The model under review builds one solid part; all positions refer to its coordinate system, in mm. A direction names the side the tool comes from. Coordinates: 2 decimals unless noted, no trailing zeros. Order: outer loops, then holes, each group sorted by start corner. A loop starts at its lowest first (then second) coordinate and runs counter-clockwise, first axis right, second up. Notation, with made-up numbers: M -2.5,87.25 L 19.5,87.25 A12 ccw 19.5,98.25 Z; hole C -24,84 d11. An arc over 180 degrees is marked long. Answer in a Markdown table with one row per item.
Autodesk Inventor part; units mm, degrees
ref_plane "YZ Plane" through (0, 0, 0) normal (1, 0, 0) x (0, 1, 0)
ref_plane "XZ Plane" through (0, 0, 0) normal (0, 1, 0) x (-1, 0, 0)
ref_plane "XY Plane" through (0, 0, 0) normal (0, 0, 1) x (1, 0, 0)
sketch "Szkic1" plane through (0, 0, 0) normal (0, 0, 1) x (1, 0, 0)
  circle A0 centre (0, 0) radius 13
  dimension "d0" = 26
extrude "Wyciągnięcie proste1" add sketch "Szkic1" along normal blind 3
sketch "Szkic2" plane through (0, 0, 3) normal (0, 0, 1) x (1, 0, 0)
  circle A0 centre (0, 0) radius 5
  dimension "d3" = 10
extrude "Wyciągnięcie proste2" add sketch "Szkic2" along normal blind 15
sketch "Szkic3" plane through (0, 0, 18) normal (0, 0, 1) x (1, 0, 0)
  circle A0 centre (0, 0) radius 4
  dimension "d6" = 8
extrude "Wyciągnięcie proste3" add sketch "Szkic3" along normal blind 50
thread "Gwint1"
sketch "Szkic4" plane through (0, 0, 68) normal (0, 0, 1) x (1, 0, 0)
  circle A0 centre (0, 0) radius 2
  dimension "d11" = 4
sketch "Szkic9" plane through (0, 0, 68) normal (0, 0, 1) x (1, 0, 0)
  circle A0 centre (0, 0) radius 4
  line L0 (-1.9365, 3.5) -> (1.9365, 3.5)
  dimension "d34" = 3.5
extrude "Wyciągnięcie proste7" cut sketch "Szkic9" against normal blind 5 contours L0 A0 picked at (-0.3981, 3.6058)
sketch "Szkic10" plane through (-1.9365, 3.5, 68) normal (0, 1, 0) x (1, 0, 0)
  line L0 (3.873, 0) -> (0, 0)
  line L1 (3.873, 5) -> (3.873, 0)
  line L2 (3.873, 5) -> (0, 5)
  line L3 (0, 0) -> (0, 5)
  line L4 (3.873, 5) -> (3.873, 0) construction
  line L5 (3.873, 2.5) -> (0, 2.5) construction
  line L6 (0, 0) -> (0, 5) construction
  point P0 (1.9365, 68)
  point P1 (1.9365, 2.5)
hole "Otwór2" at (0, 3.5, 65.5) direction (0, -1, 0) diameter 3 depth 20 tip angle 118
hole "Otwór3" at (0, 0, 68) direction (0, 0, -1) diameter 4 depth 11 tip angle 118
sketch "Szkic11" plane through (0, 0, 0) normal (0, 0, -1) x (-1, 0, 0)
  circle A0 centre (0, 0) radius 9 construction
  line L0 (9, 0) -> (-9, 0) construction
  line L1 (0, -9) -> (0, 9) construction
  dimension "d55" = 18
hole "Otwór4" at (9, 0, 0) at (-9, 0, 0) at (0, -9, 0) at (0, 9, 0) direction (0, 0, 1) diameter 4 depth 8 tip angle 118
thread "Gwint3"
thread "Gwint4"
properties part number "shaft"
(1) Take a section at D-D (z = 31.5). Write out the cut boundary in (x, y).
Report:
| item | result |
|---|---|
| outline | C 0,0 d8 |
(2) Take a section at C-C (z = 65.5). Write out the cut boundary in (x, y), then the cut area to 3 significant figures.
Report:
| item | result |
|---|---|
| outline | M -1.94,3.5 A4 ccw -1.5,-3.71 L -1.5,-1.32 A2 cw -1.5,1.32 L -1.5,3.5 Z; M 1.5,-3.71 A4 ccw 1.94,3.5 L 1.5,3.5 L 1.5,1.32 A2 cw 1.5,-1.32 Z |
| area | 24.9 mm^2 |
(3) To check wall thickness, follow line 1 (Y direction, x = 0, z = 2.15); line 2 (Z direction, x = 0, y = 2.25); line 3 (X direction, y = 0, z = 61.75). State the ranges of each line that lie inside material, in increasing order. Write a range as [from, to].
Report:
| item | result |
|---|---|
| line 1 | [-13, -11], [-7, 7], [11, 13] |
| line 2 | [0, 64], [67, 68] |
| line 3 | [-4, -2], [2, 4] |
(4) The part is to be moulded in two halves that separate along Y. For faces 1 (the conical face through (-0.34, 0.08, 56.01)), 2 (the cylindrical face through (0.9, -2.7, 64.3)), 3 (the cylindrical face through (-0.521, -3.966, 42.65)), say which applies: +Y half, -Y half, draft (parallel to the pull), parting line (faces both ways), or undercut.
Report:
| item | result |
|---|---|
| face 1 | undercut |
| face 2 | draft |
| face 3 | parting line |
(5) Machinability: for faces 4 (the flat face through (6, 0, 3)), 5 (the flat face through (0, 3.5, 67.2)), 6 (the cylindrical face through (1.2, -10.6, 1.5)), which of the approach directions +Z, -Z, +X, -X, +Y, -Y give a long, thin tool a straight path to every point of the face, cutting with its end or side? Answer none if there is none.
Report:
| item | result |
|---|---|
| face 4 | +Z |
| face 5 | +Z, +X, -X, +Y |
| face 6 | +Z, -Z |
(6) Take a section at A-A (x = -9). Write out the cut boundary in (y, z).
Report:
| item | result |
|---|---|
| outline | M -9.38,0 L -2,0 L -2,3 L -9.38,3 Z; M 2,0 L 9.38,0 L 9.38,3 L 2,3 Z |
(7) Insertion check: P1, Ø5, axis at x = 6, z = 27.5, coming from the -Y side; P2, Ø3, axis at x = 4.5, z = 43.5, coming from the +Y side; P3, Ø4.5, axis at x = 9, y = 0, coming from the +Z side. Each pin has a flat end and moves straight along its axis. Give the tip position at first contact, or say it passes through.
Report:
| item | result |
|---|---|
| P1 | y = -1.94 |
| P2 | y = 2.65 |
| P3 | z = 3 |
